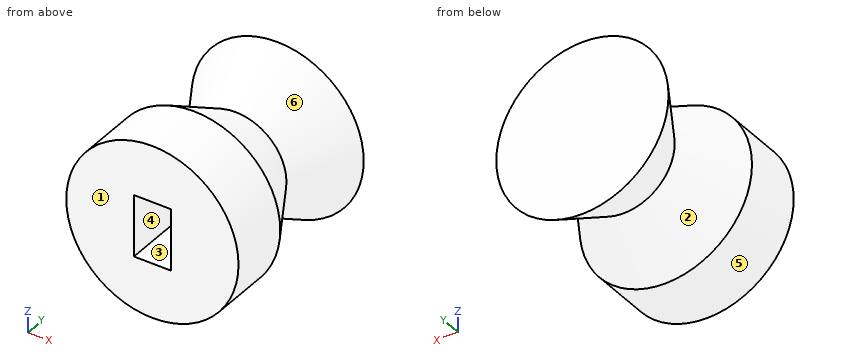
```python
from build123d import *

# Parameters (mm, degrees)
SKETCH2_R           = 7
SKETCH2_W           = 3
SKETCH2_H           = 5
BOSS_EXTRUDE1_DEPTH = 5
SKETCH3_R           = 7
BOSS_EXTRUDE2_DEPTH = 5
BOSS_EXTRUDE2_TAPER = 30
SKETCH4_R           = 4.113248654
BOSS_EXTRUDE3_DEPTH = 5
BOSS_EXTRUDE3_DRAFT = -30


with BuildPart() as part:
    # Sketch2 → Boss-Extrude1 (new body)
    with BuildSketch(Plane(origin=(0, 0, 0), x_dir=(1, 0, 0), z_dir=(0, 1, 0))):
        with Locations(Location((-3.205882353, 1.576875202, 0), (0, 0, 270))):
            Circle(SKETCH2_R)
        with Locations((-3.205882353, 1.647058824)):
            Rectangle(SKETCH2_W, SKETCH2_H, mode=Mode.SUBTRACT)
    extrude(amount=BOSS_EXTRUDE1_DEPTH)

    # Sketch3 → Boss-Extrude2 (add)
    with BuildSketch(Plane(origin=(0, 5, 0), x_dir=(1, 0, 0), z_dir=(0, 1, 0))):
        with Locations(Location((-3.205882353, 1.576875202, 0), (0, 0, 270))):
            Circle(SKETCH3_R)
    extrude(amount=BOSS_EXTRUDE2_DEPTH, taper=BOSS_EXTRUDE2_TAPER)


with BuildPart() as boss_extrude3_tool:
    # Sketch4 → Boss-Extrude3 (with draft: the straight prism first)
    with BuildSketch(Plane(origin=(0, 10, 0), x_dir=(1, 0, 0), z_dir=(0, 1, 0))):
        with Locations((-3.205882353, 1.576875202)):
            Circle(SKETCH4_R)
    extrude(amount=BOSS_EXTRUDE3_DEPTH)
    # Boss-Extrude3: the draft: its side faces are tilted about the plane it starts from
    boss_extrude3_sides = [boss_extrude3_tool.faces().sort_by_distance(p)[0] for p in [
        (-7.319131007, 12.5, -1.576875202),
    ]]
    draft(boss_extrude3_sides, Plane(origin=(0, 10, 0), x_dir=(1, 0, 0), z_dir=(0, 1, 0)), BOSS_EXTRUDE3_DRAFT)


with BuildPart() as part_1:
    add(part.part)

    # Boss-Extrude3: add boss_extrude3_tool
    add(boss_extrude3_tool.part)


solid = part_1.part
```
Work out the finished part from the listing and answer in its coordinate system (mm). Face numbers are marked on the shaded views. A direction names the side the tool comes from. Give positions to 0.01 mm unless a question says otherwise; leave off trailing zeros. Order: outer loops, then holes, each group sorted by start corner. A loop starts at its lowest first (then second) coordinate and runs counter-clockwise, first axis right, second up. Notation, with made-up numbers: M 64,35.5 L 101,35.5 A21 cw 101,62.5 Z; hole C 78.25,-30 d8. An arc over 180 degrees is marked long. Return JSON: item names as keys, results as strings.
1) A tool of negligible diameter and unlimited length cuts with its end or side. For the marked faces 5 and 6, from which of +Z, -Z, +X, -X, +Y, -Y can it reach the whole face along a straight path? Write none if from no direction.
Resolved:
{"face 5": "+Y, -Y", "face 6": "none"}
2) Straight lines are drawn through the part: line 1 along Y through (x, z) = (0.5, 0.75); line 2 along Y through (x, z) = (1.5, 2.5); line 3 along X through (y, z) = (4, 0.75). For each, find the intervals that lie inside material, in ascending order. Write a range as [from, to].
Resolved:
{"line 1": "[0, 9.55], [10.45, 15]", "line 2": "[0, 6.34], [13.66, 15]", "line 3": "[-9.81, -4.71], [-1.71, 3.4]"}
3) Each of these flat-tipped pins is pushed along its axis until it touches: pin 1 (1 mm diameter, centred on y = 3.5, z = -4.5, fed in from +X); pin 2 (3 mm diameter, centred on x = -1.5, y = 5.5, fed in from +Z); pin 3 (6 mm diameter, centred on y = 11.5, z = 0.5, fed in from -X). Where does it stop, or does it pass through?
Resolved:
{"pin 1": "x = 3.36", "pin 2": "z = 5.42", "pin 3": "x = -9.73"}
4) Section A-A, the plane y = 2.5 is taken. Write down the section's boundary in (x, z).
Resolved:
{"outline": "C -3.21,-1.58 d14; hole M -4.71,-4.15 L -1.71,-4.15 L -1.71,0.85 L -4.71,0.85 Z"}
5) For a pull along Z with two mould halves and no side action, classify the marked faces 1, 2, 3 and 4 as +Z half, -Z half, draft (parallel to the pull), parting line (faces both ways), or undercut.
Resolved:
{"face 1": "draft", "face 2": "parting line", "face 3": "undercut", "face 4": "undercut"}
6) Section C-C, the plane y = 9.25 is taken. Write down the section's boundary in (x, z).
Resolved:
{"outline": "C -3.21,-1.58 d9.09"}
7) Section B-B, the plane y = 6 is taken. Write down the section's boundary in (x, z).
Resolved:
{"outline": "C -3.21,-1.58 d12.85"}
